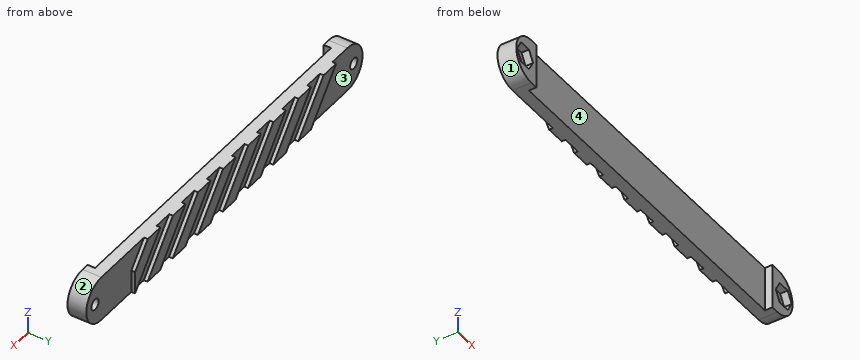
from build123d import *

# Parameters (mm, degrees)
SKETCH1_R           = 1.45
BOSS_EXTRUDE1_DEPTH = 3
BOSS_EXTRUDE2_START = 2
BOSS_EXTRUDE2_DEPTH = 2
BOSS_EXTRUDE3_DEPTH = 1


with BuildPart() as part:
    # Sketch1 → Boss-Extrude1 (new body)
    with BuildSketch(Plane(origin=(0, 0, 0), x_dir=(1, 0, 0), z_dir=(0, 1, 0))):
        with BuildLine():
            Line((-49, 6), (49, 6))
            ThreePointArc((49, 6), (55, 0), (49, -6))
            Line((49, -6), (-49, -6))
            ThreePointArc((-49, -6), (-55, 0), (-49, 6))
        make_face()
        with Locations(Location((-51.5, 0, 0), (0, 0, 270))):
            Circle(SKETCH1_R, mode=Mode.SUBTRACT)
        with Locations(Location((51.5, 0, 0), (0, 0, 270))):
            Circle(SKETCH1_R, mode=Mode.SUBTRACT)
    extrude(amount=BOSS_EXTRUDE1_DEPTH)

    # Sketch2 → Boss-Extrude2 (add)
    # profile 1 of 2: a face of its own
    with BuildSketch(Plane.XZ.offset(BOSS_EXTRUDE2_START)):
        with BuildLine():
            Line((49, 6), (47, 6))
            Line((47, 6), (47, -6))
            Line((47, -6), (49, -6))
            ThreePointArc((49, -6), (55, 0), (49, 6))
        make_face()
        Polygon((54.675426481, 0), (53.08771324, -2.75), (49.91228676, -2.75), (48.324573519, 0), (49.91228676, 2.75), (53.08771324, 2.75), align=None, mode=Mode.SUBTRACT)
    # profile 2 of 2: a face of its own
    with BuildSketch(Plane.XZ.offset(BOSS_EXTRUDE2_START)):
        with BuildLine():
            Line((-47, -6), (-47, 6))
            Line((-47, 6), (-49, 6))
            ThreePointArc((-49, 6), (-55, 0), (-49, -6))
            Line((-49, -6), (-47, -6))
        make_face()
        Polygon((-48.324573519, 0), (-49.91228676, -2.75), (-53.08771324, -2.75), (-54.675426481, 0), (-53.08771324, 2.75), (-49.91228676, 2.75), align=None, mode=Mode.SUBTRACT)
    extrude(amount=-BOSS_EXTRUDE2_DEPTH)

    # Sketch3 → Boss-Extrude3 (add)
    with BuildSketch(Plane(origin=(0, 3, 0), x_dir=(1, 0, 0), z_dir=(0, 1, 0))):
        Polygon((-32.930804426, 6), (-43, -6), (-38, -6), (-27.930804426, 6), align=None)
        Polygon((-17.930804426, 6), (-22.930804426, 6), (-33, -6), (-28, -6), align=None)
        Polygon((-7.930804426, 6), (-12.930804426, 6), (-23, -6), (-18, -6), align=None)
        Polygon((2.069195574, 6), (-2.930804426, 6), (-13, -6), (-8, -6), align=None)
        Polygon((12.069195574, 6), (7.069195574, 6), (-3, -6), (2, -6), align=None)
        Polygon((22.069195574, 6), (17.069195574, 6), (7, -6), (12, -6), align=None)
        Polygon((32.069195574, 6), (27.069195574, 6), (17, -6), (22, -6), align=None)
        Polygon((37.069195574, 6), (27, -6), (32, -6), (37.034597787, 0), align=None)
    extrude(amount=BOSS_EXTRUDE3_DEPTH)


solid = part.part
Design review of the part built by this model. Coordinates are the model's own, in mm. Face numbers are marked on the shaded views. Coordinates: 2 decimals unless noted, no trailing zeros. Order: outer loops, then holes, each group sorted by start corner. A loop starts at its lowest first (then second) coordinate and runs counter-clockwise, first axis right, second up. Notation, with made-up numbers: M 4.25,6.5 L 41.25,6.5 A17 ccw 41.25,29.5 Z; hole C 6.5,34 d1. An arc over 180 degrees is marked long. Use a Markdown table: item, result.
(1) Add section C-C (x = 35). Give the boundary of the cut face in (y, z), then the cut area to 3 significant figures.
Worked answers:
| item | result |
|---|---|
| outline | M 0,-6 L 3,-6 L 3,-3.53 L 4,-3.53 L 4,2.42 L 3,2.42 L 3,6 L 0,6 Z |
| area | 42.0 mm2 |
(2) Wall thickness on probe 1 along X at (y, z) = (1.9, 0); probe 2 along Y at (x, z) = (-21.5, -0.75); probe 3 along Y at (x, z) = (16, -1.5): over which ranges is each line inside the solid? List them lowest first.
Worked answers:
| item | result |
|---|---|
| probe 1 | x = -55 to -52.95, -50.05 to 50.05, 52.95 to 55 |
| probe 2 | y = 0 to 3 |
| probe 3 | y = 0 to 4 |
(3) Add section B-B (y = 1.75). Give the boundary of the cut face in (x, z).
Worked answers:
| item | result |
|---|---|
| outline | M -49,-6 L 49,-6 A6 ccw 49,6 L -49,6 A6 ccw Z; hole C -51.5,0 d2.9; hole C 51.5,0 d2.9 |
(4) For P1, Ø1, axis at x = 51.5, y = -1, coming from the -Z side; P2, Ø3.5, axis at x = -51.5, z = 0, coming from the -Y side; P3, Ø1.6, axis at x = 52, y = -1, coming from the +Z side, all flat-tipped, find the tip position at first contact; note any pin that passes through.
Worked answers:
| item | result |
|---|---|
| P1 | stops at z = -5.66 |
| P2 | stops at y = 0 |
| P3 | stops at z = 5.58 |
(5) Add section A-A (x = 51.5). Give the boundary of the cut face in (y, z).
Worked answers:
| item | result |
|---|---|
| outline | M -2,-5.45 L 3,-5.45 L 3,-1.45 L 0,-1.45 L 0,-2.75 L -2,-2.75 Z; M -2,2.75 L 0,2.75 L 0,1.45 L 3,1.45 L 3,5.45 L -2,5.45 Z |
(6) Draft analysis for pull direction X (two halves, no side actions). For the marked faces 1, 2, 3 and 4, state which applies: released by +X, released by -X, zero draft, split by the parting line, or undercut.
Worked answers:
| item | result |
|---|---|
| face 1 | released by -X |
| face 2 | released by +X |
| face 3 | zero draft |
| face 4 | undercut |
